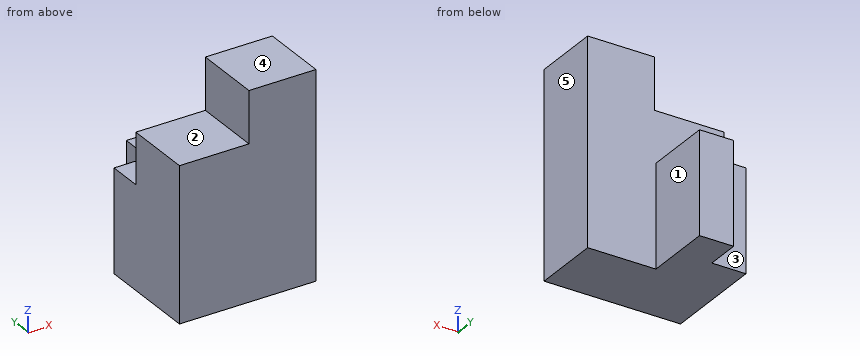
from build123d import *

# Parameters (mm, degrees)
SKETCH1_W           = 40
SKETCH1_H           = 40
BOSS_EXTRUDE1_DEPTH = 60
SKETCH2_W           = 20
SKETCH2_H           = 60
CUT_EXTRUDE1_DEPTH  = 20
SKETCH3_W           = 10
SKETCH3_H           = 30
CUT_EXTRUDE2_DEPTH  = 10
SKETCH4_W           = 20
SKETCH4_H           = 30
CUT_EXTRUDE3_DEPTH  = 20
SKETCH5_W           = 20.369010991
SKETCH5_H           = 15.116556711
CUT_EXTRUDE4_DEPTH  = 20


with BuildPart() as part:
    # Sketch1 → Boss-Extrude1 (new body)
    with BuildSketch(Plane.XY):
        with Locations((20, 20)):
            Rectangle(SKETCH1_W, SKETCH1_H)
    extrude(amount=BOSS_EXTRUDE1_DEPTH)

    # Sketch2 → Cut-Extrude1 (cut)
    with BuildSketch(Plane(origin=(0, 40, 0), x_dir=(1, 0, 0), z_dir=(0, 1, 0))):
        with Locations((30, -30)):
            Rectangle(SKETCH2_W, SKETCH2_H)
    extrude(amount=-CUT_EXTRUDE1_DEPTH, mode=Mode.SUBTRACT)

    # Sketch3 → Cut-Extrude2 (cut)
    with BuildSketch(Plane(origin=(0, 40, 0), x_dir=(1, 0, 0), z_dir=(0, 1, 0))):
        with Locations((5, -15)):
            Rectangle(SKETCH3_W, SKETCH3_H)
    extrude(amount=-CUT_EXTRUDE2_DEPTH, mode=Mode.SUBTRACT)

    # Sketch4 → Cut-Extrude3 (cut)
    with BuildSketch(Plane(origin=(0, 40, 0), x_dir=(1, 0, 0), z_dir=(0, 1, 0))):
        with Locations((10, -45)):
            Rectangle(SKETCH4_W, SKETCH4_H)
    extrude(amount=-CUT_EXTRUDE3_DEPTH, mode=Mode.SUBTRACT)

    # Sketch5 → Cut-Extrude4 (cut)
    with BuildSketch(Plane(origin=(0, 20, 0), x_dir=(1, 0, 0), z_dir=(0, 1, 0))):
        with Locations((10.184505495, -52.441721645)):
            Rectangle(SKETCH5_W, SKETCH5_H)
    extrude(amount=-CUT_EXTRUDE4_DEPTH, mode=Mode.SUBTRACT)


solid = part.part
Design review of the part built by this model. Coordinates are the model's own, in mm. Face numbers are marked on the shaded views. A direction names the side the tool comes from. Round coordinates to 2 decimals unless told otherwise and drop trailing zeros. Write each loop counter-clockwise with the first axis right and the second up, starting at its lowest first coordinate (ties: lowest second). Pieces come first, ordered by that corner, then holes. Notation, with made-up numbers: (5, 18) - (59, 18) arc R26 cw to (59, 51) - close; hole circle Ø2 at (57, -13). An arc over 180 degrees is marked (long way). Use a Markdown table: item, result. Add a question column.
1. Clearance check with flat-ended pins moving along their axes: pin 1 (10 mm diameter, centred on x = 12, y = 15, fed in from +Z); pin 2 (3 mm diameter, centred on y = 35.5, z = 12.5, fed in from -X); pin 3 (6 mm diameter, centred on x = 13, y = 30, fed in from +Z). State where each tip first meets the part, or that it passes through.
2. Wall thickness on probe 1 along X at (y, z) = (32, 5); probe 2 along Z at (x, y) = (18, 13.5); probe 3 along Y at (x, z) = (3.5, 13): over which ranges is each line inside the solid? List them lowest first.
3. We need section B-B (y = 21). State the section outline as (x, z) points.
4. For the marked faces 1, 2, 3, 4 and 5, list the 3-axis set-ups (+Z, -Z, +X, -X, +Y, -Y) from which the entire face can be reached by the end or side of a thin tool; tool diameter is ignored.
5. We need section D-D (y = 16.5). State the section outline as (x, z) points, then the cut area to 3 significant figures.
6. We need section C-C (x = 11.5). State the section outline as (y, z) points.
7. We need section A-A (z = 9). State the section outline as (x, y) points.
Output:
| question | item | result |
|---|---|---|
| 1 | pin 1 | stops at z = 44.88 |
| 1 | pin 2 | stops at x = 10 |
| 1 | pin 3 | stops at z = 30 |
| 2 | probe 1 | x = 10 to 20 |
| 2 | probe 2 | z = 0 to 44.88 |
| 2 | probe 3 | y = 0 to 30 |
| 3 | outline | (0, 0) - (20, 0) - (20, 30) - (0, 30) - close |
| 4 | face 1 | +Z, -Z, +X, +Y |
| 4 | face 2 | +Z, -X, +Y, -Y |
| 4 | face 3 | +Z, -Z, -X, +Y |
| 4 | face 4 | +Z, +X, -X, +Y, -Y |
| 4 | face 5 | +Z, -Z, +X, +Y, -Y |
| 5 | outline | (0, 0) - (40, 0) - (40, 60) - (20.37, 60) - (20.37, 44.88) - (0, 44.88) - close |
| 5 | area | 2,090 mm2 |
| 6 | outline | (0, 0) - (40, 0) - (40, 30) - (20, 30) - (20, 44.88) - (0, 44.88) - close |
| 7 | outline | (0, 0) - (40, 0) - (40, 20) - (20, 20) - (20, 40) - (10, 40) - (10, 30) - (0, 30) - close |
